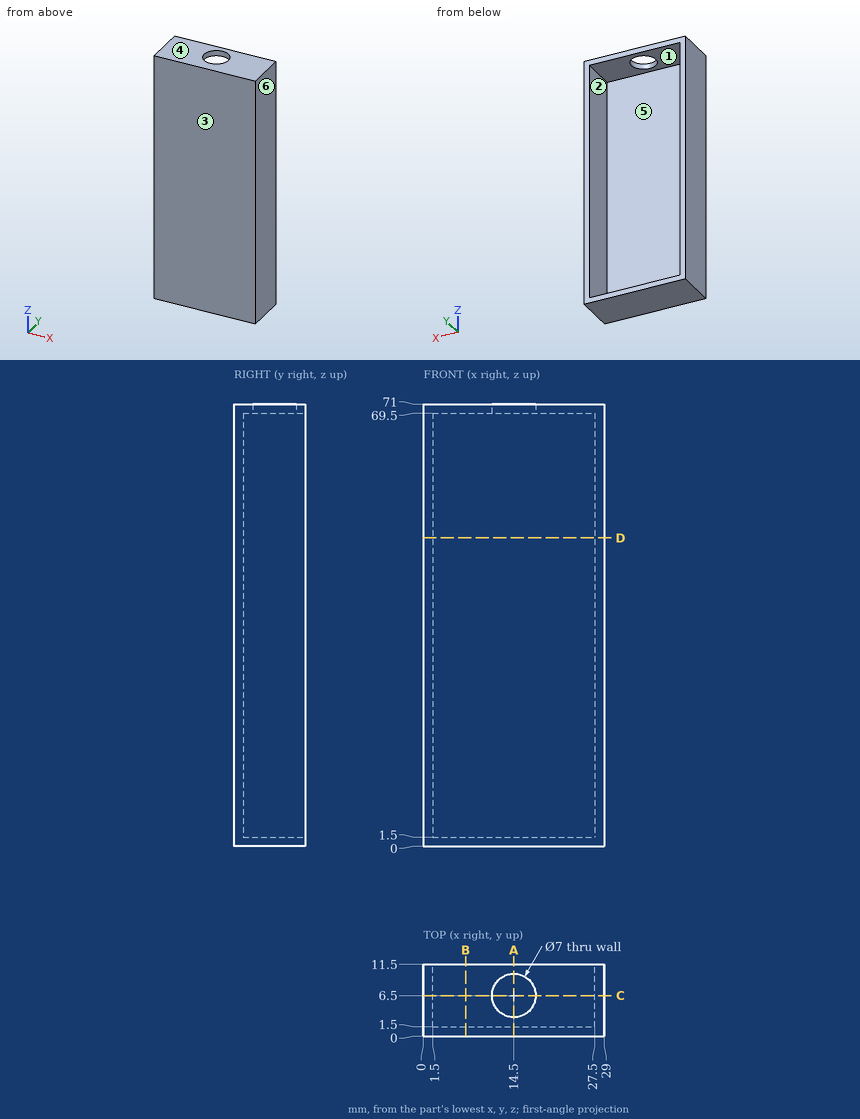
Study the drawing (mm; zero at the part's minimum x, y, z) and answer. A direction names the side the tool comes from. Coordinates: 2 decimals unless noted, no trailing zeros. Write each loop counter-clockwise with the first axis right and the second up, starting at its lowest first coordinate (ties: lowest second). Pieces come first, ordered by that corner, then holes.
Q1. A cutting plane is placed at D-D, the plane z = 49.5. Give the vertices of the cut face in (x, y).
Q2. A cutting plane is placed at B-B, the plane x = 6.75. Give the vertices of the cut face in (y, z), then the cut area to 4 significant figures.
Q3. Which of the six approach directions +Z, -Z, +X, -X, +Y, -Y give full straight-line access (tool end or side, diameter ignored) to the marked faces 5 and 6?
Q4. A cutting plane is placed at C-C, the plane y = 6.5. Give the vertices of the cut face in (x, z).
Q5. A cutting plane is placed at A-A, the plane x = 14.5. Give the vertices of the cut face in (y, z).
Q6. Determine the mould class of the marked faces 1, 2, 3 and 4 for opening direction Z: released by +Z, released by -Z, zero draft, split by the parting line, or undercut.
Q7. Find the intervals of material crossed by line 1 (X direction, y = 10, z = 44); line 2 (Z direction, x = 22.5, y = 5.5); line 3 (Y direction, x = 14.5, z = 70.15), in increasing order.
Q8. This flat-tipped pin is pushed along its axis until it touches: pin 1 Ø2 at (x, z) = (13.5, 18.5) entering from +Y. Where does it stop, or does it pass through?
Findings below:
1. outline: (0, 0) - (29, 0) - (29, 11.5) - (27.5, 11.5) - (27.5, 1.5) - (1.5, 1.5) - (1.5, 11.5) - (0, 11.5) - close
2. outline: (0, 0) - (11.5, 0) - (11.5, 1.5) - (1.5, 1.5) - (1.5, 69.5) - (11.5, 69.5) - (11.5, 71) - (0, 71) - close
2. area: 136.5 mm2
3. face 5: +Y
3. face 6: +Z, -Z, +X, +Y, -Y
4. outline: (0, 0) - (29, 0) - (29, 71) - (18, 71) - (18, 69.5) - (27.5, 69.5) - (27.5, 1.5) - (1.5, 1.5) - (1.5, 69.5) - (11, 69.5) - (11, 71) - (0, 71) - close
5. outline: (0, 0) - (11.5, 0) - (11.5, 1.5) - (1.5, 1.5) - (1.5, 69.5) - (3, 69.5) - (3, 71) - (0, 71) - close; (10, 69.5) - (11.5, 69.5) - (11.5, 71) - (10, 71) - close
6. face 1: undercut
6. face 2: undercut
6. face 3: zero draft
6. face 4: released by +Z
7. line 1: x = 0 to 1.5, 27.5 to 29
7. line 2: z = 0 to 1.5, 69.5 to 71
7. line 3: y = 0 to 3, 10 to 11.5
8. pin 1: stops at y = 1.5
